Model file for the job. Use its own axes, mm. A direction names the side the tool comes from. Give positions to 0.01 mm unless a question says otherwise; leave off trailing zeros. Write each loop counter-clockwise with the first axis right and the second up, starting at its lowest first coordinate (ties: lowest second). Pieces come first, ordered by that corner, then holes.
Autodesk Inventor part; units mm, degrees
ref_plane "YZ Plane" through (0, 0, 0) normal (1, 0, 0) x (0, 1, 0)
ref_plane "XZ Plane" through (0, 0, 0) normal (0, 1, 0) x (-1, 0, 0)
ref_plane "XY Plane" through (0, 0, 0) normal (0, 0, 1) x (1, 0, 0)
sketch "Эскиз1" plane through (0, 0, 0) normal (1, 0, 0) x (0, 1, 0)
  line L0 (-17, 21) -> (17, 21)
  line L1 (21, 17) -> (21, -17)
  line L2 (17, -21) -> (-17, -21)
  line L3 (-21, -17) -> (-21, 17)
  line L4 (-21, 21) -> (21, -21) construction
  line L5 (21, 21) -> (-21, -21) construction
  line L6 (21, 17) -> (17, 21)
  line L7 (21, -17) -> (17, -21)
  line L8 (-17, 21) -> (-21, 17)
  line L9 (-21, -17) -> (-17, -21)
  point P0 (0, 0)
  dimension "d0" = 42
  dimension "d1" = 42
  dimension "d2" = 4
  dimension "d3" = 4
  dimension "d4" = 4
  dimension "d5" = 4
  dimension "d6" = 4
  dimension "d7" = 4
  dimension "d8" = 4
  dimension "d9" = 4
extrude "Выдавливание1" add sketch "Эскиз1" against normal blind 40
ref_plane "РабПлоскость1" through (-8, 0, 0) normal (1, 0, 0) x (0, 0, -1)
sketch "Эскиз2" plane through (-8, 0, 0) normal (1, 0, 0) x (0, 0, -1)
  line L0 (-21, -17) -> (-17, -21)
  line L1 (-14, -21) -> (14, -21)
  line L2 (17, -21) -> (21, -17)
  line L3 (21, -14) -> (21, 14)
  line L4 (21, 17) -> (17, 21)
  line L5 (17, 21) -> (-14, 21)
  line L6 (-17, 21) -> (-21, 17)
  line L7 (-21, 14) -> (-21, -14)
  line L8 (14, 21) -> (-17, 21)
  line L9 (-21, -17) -> (-21, 17)
  line L10 (21, -17) -> (21, 17)
  line L11 (-17, -21) -> (17, -21)
  line L12 (-14, 21) -> (-21, 14)
  line L13 (-21, -14) -> (-14, -21)
  line L14 (21, -14) -> (14, -21)
  line L15 (21, 14) -> (14, 21)
  point P0 (0, 0)
  point P1 (-21, 21)
  point P2 (-21, -21)
  point P3 (21, -21)
  point P4 (21, 21)
  point P5 (14, -21)
  point P6 (-14, 21)
  dimension "d14" = 7
  dimension "d15" = 7
  dimension "d16" = 7
  dimension "d17" = 7
  dimension "d18" = 7
  dimension "d19" = 7
  dimension "d20" = 7
  dimension "d21" = 7
extrude "Выдавливание2" cut sketch "Эскиз2" against normal blind 23 contours L9 L13 L11 L0 | L9 L6 L8 L12 | L14 L10 L2 L11 | L5 L4 L10 L15
sketch "Эскиз3" plane through (0, 0, 0) normal (1, 0, 0) x (0, 0, -1)
  line L0 (-21, -17) -> (-17, -21)
  line L1 (-17, -21) -> (17, -21)
  line L2 (17, -21) -> (21, -17)
  line L3 (21, -17) -> (21, 17)
  line L4 (21, 17) -> (17, 21)
  line L5 (17, 21) -> (-17, 21)
  line L6 (-17, 21) -> (-21, 17)
  line L7 (-21, 17) -> (-21, -17)
  circle A0 centre (0, 0) radius 2.5
  dimension "d24" = 5
extrude "Выдавливание3" add sketch "Эскиз3" along normal blind 15 contours A0
sketch "Эскиз4" plane through (0, 0, 0) normal (1, 0, 0) x (0, 0, -1)
  line L0 (-15.5, -15.5) -> (15.5, -15.5)
  line L1 (15.5, -15.5) -> (15.5, 15.5)
  line L2 (15.5, 15.5) -> (-15.5, 15.5)
  line L3 (-15.5, 15.5) -> (-15.5, -15.5)
  line L4 (-15.5, -15.5) -> (15.5, 15.5) construction
  line L5 (15.5, -15.5) -> (-15.5, 15.5) construction
  circle A0 centre (-15.5, 15.5) radius 1.5
  circle A1 centre (15.5, 15.5) radius 1.5
  circle A2 centre (15.5, -15.5) radius 1.5
  circle A3 centre (-15.5, -15.5) radius 1.5
  point P0 (0, 0)
  dimension "d27" = 31
  dimension "d28" = 31
  dimension "d29" = 3
  dimension "d30" = 3
  dimension "d31" = 3
  dimension "d32" = 3
extrude "Выдавливание4" cut sketch "Эскиз4" against normal blind 8 contours L3 A3 L0 | L0 A3 L3 | A2 L1 L0 | L0 L1 A2 | A0 L2 L3 | L3 L2 A0 | A1 L2 L1 | L1 L2 A1
sketch "Эскиз5" plane through (15, 0, 0) normal (1, 0, 0) x (0, 0, -1)
  point P0 (0, 0)
sketch "Эскиз6" plane through (0, 0, 0) normal (1, 0, 0) x (0, 0, -1)
  circle A0 centre (0, 0) radius 2.5
  circle A1 centre (0, 0) radius 11
  circle A2 centre (0, 0) radius 5
  dimension "d35" = 22
  dimension "d36" = 6
extrude "Выдавливание5" add sketch "Эскиз6" along normal blind 2 contours A1
equation "\"d3\" = d2"
equation "\"d4\" = d2"
equation "\"d5\" = d4"
equation "\"d6\" = d2"
equation "\"d7\" = d6"
equation "\"d8\" = d2"
equation "\"d9\" = d8"
properties part number "Шаговик17" material "Сталь, литейная"
1. Slice it at D-D, the plane x = -23. Write the cut outline in (y, z), and give its area (3 significant figures).
Calculated:
outline: (-21, -14) - (-14, -21) - (14, -21) - (21, -14) - (21, 14) - (14, 21) - (-14, 21) - (-21, 14) - close
area: 1,670 mm2
2. Probe probe 1 along Z at (x, y) = (-2, 15.5); probe 2 along Z at (x, y) = (-6, -15). List the from-to ranges inside material, lowest first.
Calculated:
probe 1: z = -21 to -17, -14 to 14, 17 to 21
probe 2: z = -21 to -16.91, -14.09 to 14.09, 16.91 to 21
3. Slice it at A-A, the plane x = -1.5. Write the cut outline in (y, z), and give its area (3 significant figures).
Calculated:
outline: (-21, -17) - (-17, -21) - (17, -21) - (21, -17) - (21, 17) - (17, 21) - (-17, 21) - (-21, 17) - close; hole circle Ø3 at (-15.5, -15.5); hole circle Ø3 at (-15.5, 15.5); hole circle Ø3 at (15.5, -15.5); hole circle Ø3 at (15.5, 15.5)
area: 1,700 mm2
4. Pin check, flat tips, straight feed: P1, Ø0.9, axis at y = -15, z = -15, coming from the +X side; P2, Ø5.5, axis at y = -17, z = 19, coming from the +X side. Stop position of each tip, or through.
Calculated:
P1: stops at x = -8
P2: stops at x = 0
5. Slice it at B-B, the plane z = 0. Write the cut outline in (x, y).
Calculated:
outline: (-40, -21) - (0, -21) - (0, -11) - (2, -11) - (2, -5) - (0, -5) - (0, -2.5) - (15, -2.5) - (15, 2.5) - (0, 2.5) - (0, 5) - (2, 5) - (2, 11) - (0, 11) - (0, 21) - (-40, 21) - close
6. Pull direction X, two halves, no side cores. Call faces 6 (the flat face through (-31, -18, 18)), 7 (the cylindrical face through (-3.94, -15.43, 17)), 8 (the flat face through (0, 2, -2)): +X half, -X half, draft (parallel to the pull), parting line (faces both ways), or undercut.
Calculated:
face 6: undercut
face 7: draft
face 8: +X half
7. Which spindle directions (+Z, -Z, +X, -X, +Y, -Y) get a long thin tool onto all of the face, cutting with end or side? Do faces 1 (the flat face through (0, -10, 10)), 2 (the flat face through (-19, -17, -18)), 3 (the flat face through (-8, -18, 18)), 4 (the flat face through (-8, 18, -18)), 5 (the flat face through (-19, 18, 17)). Say none if no direction does.
Calculated:
face 1: +X
face 2: -Z, -Y
face 3: +Z, -Y
face 4: -Z, +Y
face 5: +Z, +Y
